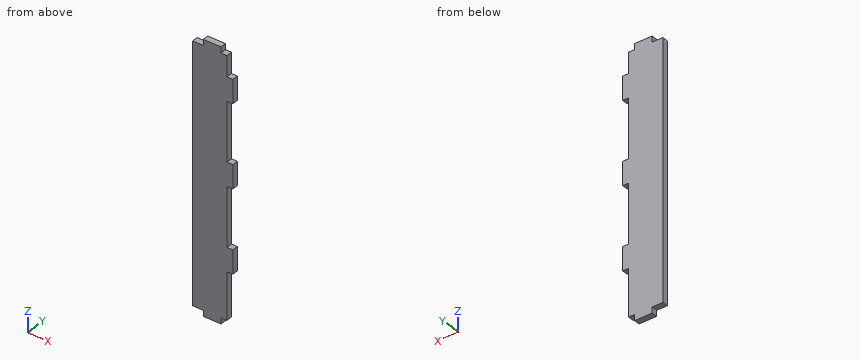
Autodesk Inventor part; units mm, degrees
ref_plane "YZ Plane" through (0, 0, 0) normal (1, 0, 0) x (0, 1, 0)
ref_plane "XZ Plane" through (0, 0, 0) normal (0, 1, 0) x (-1, 0, 0)
ref_plane "XY Plane" through (0, 0, 0) normal (0, 0, 1) x (1, 0, 0)
sketch "Sketch1" plane through (0, 0, 0) normal (0, 1, 0) x (-1, 0, 0)
  line L0 (-14.5, 108.75) -> (14.5, 108.75)
  line L1 (14.5, 108.75) -> (14.5, -108.75)
  line L2 (14.5, -108.75) -> (-14.5, -108.75)
  line L3 (-14.5, -108.75) -> (-14.5, 108.75)
  line L4 (-14.5, 108.75) -> (14.5, -108.75) construction
  line L5 (14.5, 108.75) -> (-14.5, -108.75) construction
  line L6 (-14.5, 91.25) -> (-19.5, 91.25)
  line L7 (-19.5, 91.25) -> (-19.5, 71.25)
  line L8 (-19.5, 71.25) -> (-14.5, 71.25)
  line L9 (-14.5, 71.25) -> (-14.5, 91.25)
  line L10 (-14.5, 21.25) -> (-19.5, 21.25)
  line L11 (-19.5, 21.25) -> (-19.5, 1.25)
  line L12 (-19.5, 1.25) -> (-14.5, 1.25)
  line L13 (-14.5, 1.25) -> (-14.5, 21.25)
  line L14 (-14.5, -48.75) -> (-19.5, -48.75)
  line L15 (-19.5, -48.75) -> (-19.5, -68.75)
  line L16 (-19.5, -68.75) -> (-14.5, -68.75)
  line L17 (-14.5, -68.75) -> (-14.5, -48.75)
  line L18 (5.5, 108.75) -> (-9.5, 108.75)
  line L19 (-9.5, 108.75) -> (-9.5, 113.75)
  line L20 (-9.5, 113.75) -> (5.5, 113.75)
  line L21 (5.5, 113.75) -> (5.5, 108.75)
  line L22 (5.5, -108.75) -> (-9.5, -108.75)
  line L23 (-9.5, -108.75) -> (-9.5, -113.75)
  line L24 (-9.5, -113.75) -> (5.5, -113.75)
  line L25 (5.5, -113.75) -> (5.5, -108.75)
  point P0 (0, 0)
  point P1 (-14.5, 71.25)
  point P2 (-14.5, 1.25)
  point P3 (-14.5, -68.75)
  dimension "d0" = 29
  dimension "d2" = 5
  dimension "d3" = 20
  dimension "d4" = 20
  dimension "d5" = 20
  dimension "d6" = 50
  dimension "d7" = 50
  dimension "d8" = 17.5
  dimension "d10" = 15
  dimension "d11" = 9
  dimension "d14" = 5
  dimension "d15" = 40
  dimension "d16" = 15
  dimension "d17" = 5
  dimension "d18" = 9
extrude "Extrusion1" add sketch "Sketch1" along normal blind 5
equation "\"BendRadius\" = Thickness"
equation "\"BendReliefWidth\" = Thickness"
equation "\"BendReliefDepth\" = 0.5 * Thickness"
equation "\"CornerReliefSize\" = 4 * Thickness"
equation "\"MinimumRemnant\" = 2 * Thickness"
equation "\"TransitionRadius\" = BendRadius"
equation "\"JacobiRadiusSize\" = BendRadius"
equation "\"GapSize\" = Thickness"
properties part number "Manija1"
Part model, mm, in its own coordinate system. Round coordinates to 2 decimals unless told otherwise and drop trailing zeros. Order: outer loops, then holes, each group sorted by start corner. A loop starts at its lowest first (then second) coordinate and runs counter-clockwise, first axis right, second up. Notation, with made-up numbers: (53, 67.5) -> (100, 67.5) arc R21 cw to (100, 88.5) -> close; hole circle Ø2 at (52, 60.25). An arc over 180 degrees is marked (long way). Put each result on its own line as item: value.
Q1. Pin check, flat tips, straight feed: pin 1 Ø1.5 at (y, z) = (1.5, 112.5) entering from -X; pin 2 Ø2.5 at (x, y) = (17.5, 2.5) entering from +Z; pin 3 Ø2.5 at (x, y) = (11.5, 1.5) entering from +Z; pin 4 Ø1.5 at (x, z) = (13.5, 44.5) entering from -Y. Stop position of each tip, or through.
From the geometry:
pin 1: stops at x = -5.5
pin 2: stops at z = 91.25
pin 3: stops at z = 108.75
pin 4: stops at y = 0
Q2. Band-saw the part on B-B (x = -7.5). Give the cut face in (y, z), and give its area (3 significant figures).
From the geometry:
outline: (0, -108.75) -> (5, -108.75) -> (5, 108.75) -> (0, 108.75) -> close
area: 1,090 mm2
Q3. Wall check: line 1 (Z direction, x = 17, y = 2.45); line 2 (Z direction, x = -12, y = 4.7); line 3 (X direction, y = 4, z = 25). Give the ranges that are in metal, low to high. Write a range as [from, to].
From the geometry:
line 1: z = [-68.75, -48.75], [1.25, 21.25], [71.25, 91.25]
line 2: z = [-108.75, 108.75]
line 3: x = [-14.5, 14.5]
Q4. Band-saw the part on C-C (z = 53.5). Give the cut face in (x, y), and give its area (3 significant figures).
From the geometry:
outline: (-14.5, 0) -> (14.5, 0) -> (14.5, 5) -> (-14.5, 5) -> close
area: 145 mm2
Q5. Band-saw the part on A-A (y = 3.5). Give the cut face in (x, z).
From the geometry:
outline: (-14.5, -108.75) -> (-5.5, -108.75) -> (-5.5, -113.75) -> (9.5, -113.75) -> (9.5, -108.75) -> (14.5, -108.75) -> (14.5, -68.75) -> (19.5, -68.75) -> (19.5, -48.75) -> (14.5, -48.75) -> (14.5, 1.25) -> (19.5, 1.25) -> (19.5, 21.25) -> (14.5, 21.25) -> (14.5, 71.25) -> (19.5, 71.25) -> (19.5, 91.25) -> (14.5, 91.25) -> (14.5, 108.75) -> (9.5, 108.75) -> (9.5, 113.75) -> (-5.5, 113.75) -> (-5.5, 108.75) -> (-14.5, 108.75) -> close
